Part print with two shaded views. Sizes in mm from the minimum x, y, z corner. A direction names the side the tool comes from. Coordinates: 2 decimals unless noted, no trailing zeros. Write each loop counter-clockwise with the first axis right and the second up, starting at its lowest first coordinate (ties: lowest second). Pieces come first, ordered by that corner, then holes. Notation, with made-up numbers: M 35,-0.75 L 72,-0.75 A14 ccw 72,23.25 Z; hole C 79,57.5 d10. An arc over 180 degrees is marked long. Use CSV: the item, a comma, the result in double quotes. Start each with the question number.
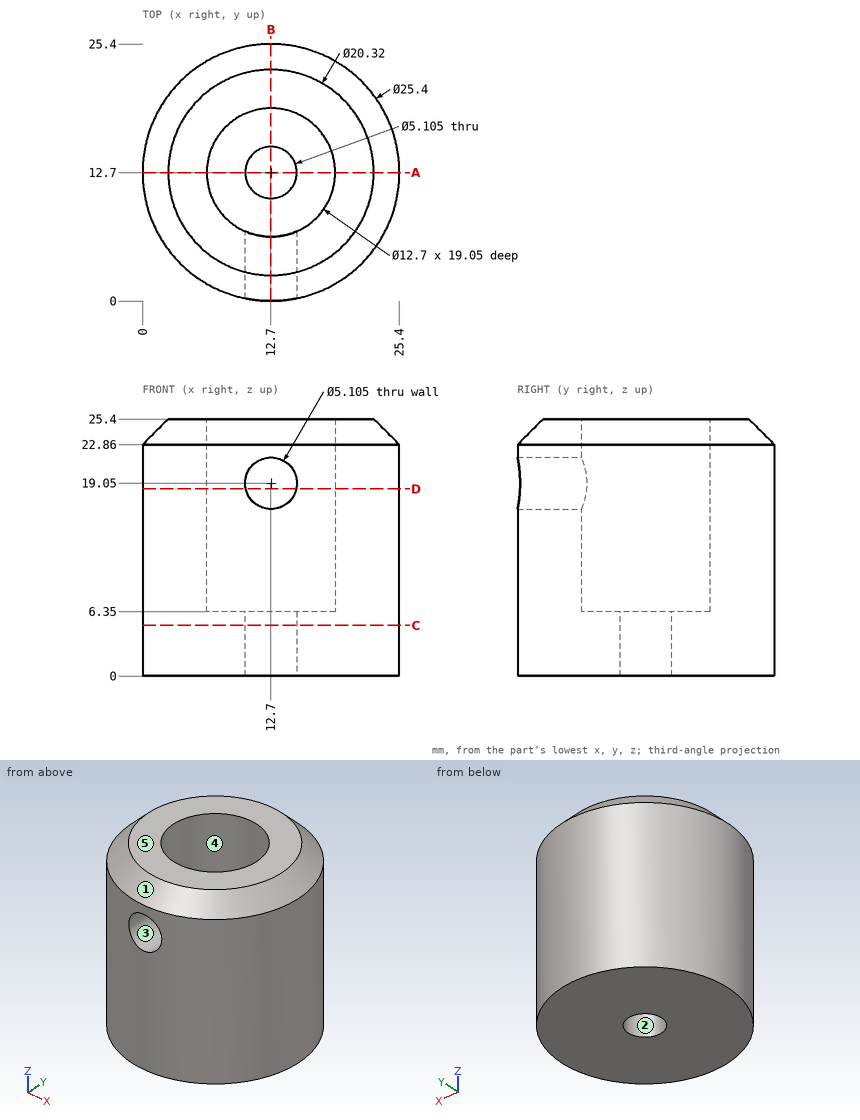
1. 3-axis set-ups, long thin cutter, end or side, ignore diameter. For the marked faces 4 and 5: which of +Z, -Z, +X, -X, +Y, -Y reach the whole face in a straight line?
2. Slice it at C-C (z = 5). List the corners of the cut face in (x, y) (1 decimal).
3. Slice it at B-B (x = 12.7). List the corners of the cut face in (y, z), and give its area (3 significant figures).
4. Slice it at A-A (y = 12.7). List the corners of the cut face in (x, z).
5. Slice it at D-D (z = 18.5). List the corners of the cut face in (x, y).
6. Pull direction Z, two halves, no side cores. Call the marked faces 1, 2 and 3: pulls with the +Z half, pulls with the -Z half, needs draft (parallel to the pull), parting line crosses it, or undercut.
7. Drill centre lines: line 1 along Y through (x, z) = (12.7, 3); line 2 along Z through (x, y) = (12.75, 16.75); line 3 along X through (y, z) = (11.25, 5.75). Where is each one in solid material? Low to high. Write a range as from..to.
8. Flat gauge pins, fed straight in: pin 1 (4 mm diameter, centred on x = 8, z = 16.5, fed in from -Y); pin 2 (4 mm diameter, centred on x = 12.7, z = 19.05, fed in from -Y); pin 3 (3 mm diameter, centred on x = 4, z = 16.5, fed in from +Y). Where does each tip first touch, or does it go through?
Established:
1,face 4,"+Z"
1,face 5,"+Z, +X, -X, +Y, -Y"
2,outline,"C 12.7,12.7 d25.4; hole C 12.7,12.7 d5.1"
3,outline,"M 0,0 L 10.15,0 L 10.15,6.35 L 6.35,6.35 L 6.35,16.5 L 0,16.5 Z; M 0,21.6 L 6.35,21.6 L 6.35,25.4 L 2.54,25.4 L 0,22.86 Z; M 15.25,0 L 25.4,0 L 25.4,22.86 L 22.86,25.4 L 19.05,25.4 L 19.05,6.35 L 15.25,6.35 Z"
3,area,"332 mm2"
4,outline,"M 0,0 L 10.15,0 L 10.15,6.35 L 6.35,6.35 L 6.35,25.4 L 2.54,25.4 L 0,22.86 Z; M 15.25,0 L 25.4,0 L 25.4,22.86 L 22.86,25.4 L 19.05,25.4 L 19.05,6.35 L 15.25,6.35 Z"
5,outline,"M 10.21,0.25 L 10.21,6.86 A6.35 cw long 15.19,6.86 L 15.19,0.25 A12.7 ccw long Z"
6,face 1,"pulls with the +Z half"
6,face 2,"needs draft"
6,face 3,"undercut"
7,line 1,"y = 0..10.15, 15.25..25.4"
7,line 2,"z = 0..6.35"
7,line 3,"x = 0.08..10.6, 14.8..25.32"
8,pin 1,"stops at y = 0.29"
8,pin 2,"stops at y = 18.73"
8,pin 3,"stops at y = 23.16"
